Input: part model. Units: mm. Frame: model coordinates. Face numbers are marked on the shaded views. A direction names the side the tool comes from. Coordinates: 2 decimals unless noted, no trailing zeros. Loops run counter-clockwise (first coordinate to the right, second up) from the corner with the lowest first, then second, coordinate; pieces in that order, holes last. Notation, with made-up numbers: (5.5, 41) -> (27.5, 41) arc R26 ccw to (27.5, 73) -> close; hole circle Ø1 at (84.25, -18.75). An arc over 180 degrees is marked (long way). Put each result on its own line as item: value. Start each with the question number.
1) Pull-direction query (Y, two-part tool) for the marked faces 4, 5, 6 and 7; classes: pulls with the +Y half, pulls with the -Y half, needs draft (parallel to the pull), parting line crosses it, or undercut.
2) Cut plane D-D (z = 28). Return the cut outline in (x, y), plus the area to 3 significant figures.
3) Cut plane B-B (x = 0). Return the cut outline in (y, z).
4) Material intervals for L1, parallel to X at y = -2.5, z = 12; L2, parallel to Y at x = 0, z = 4.5; L3, parallel to Z at x = -4.5, y = 9.5, sorted ascending.
5) Set-up query: the marked faces 1, 2 and 3. Return all of +Z, -Z, +X, -X, +Y, -Y with unobstructed straight access to the full face (end or side cutting, diameter ignored); none if empty.
6) Cut plane A-A (z = 22). Return the cut outline in (x, y), plus the area to 3 significant figures.
7) Contact query for flat-ended pins moving along their axis: P1, Ø9, axis at y = 0, z = 32, coming from the -X side; P2, Ø13.5, axis at x = -20.5, z = 21, coming from the -Y side; P3, Ø2, axis at x = 14.5, y = 9.5, coming from the +Z side; P4, Ø2, axis at x = 23, y = -2.5, coming from the +Z side. Output: stop coordinate, or through.
8) Cut plane C-C (y = 6). Return the cut outline in (x, z).
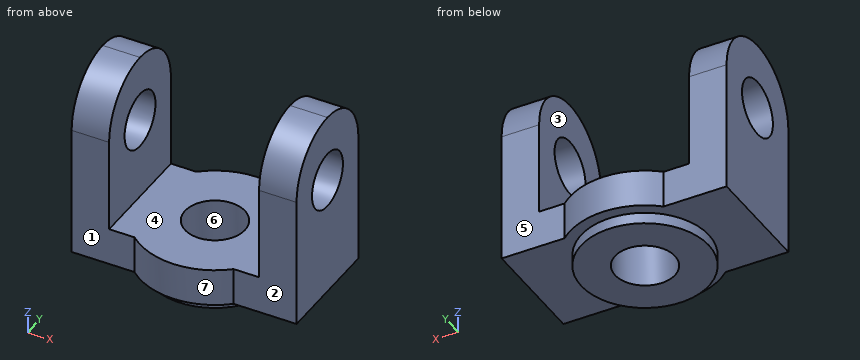
from build123d import *

# Parameters (mm, degrees)
F0_R     = 20
F0_R_2   = 8
F1_DEPTH = 10
F2_R     = 17
F2_R_2   = 8
F3_DEPTH = 3
F5_DEPTH = 15
F6_R     = 8
F7_DEPTH = 25
F8_R     = 7.5
F9_DEPTH = 30


with BuildPart() as f1:
    # F0 (on Top) → F1 (new body)
    with BuildSketch(Plane.XY):
        Circle(F0_R)
        Circle(F0_R_2, mode=Mode.SUBTRACT)
    extrude(amount=F1_DEPTH)

    # F2 (on Top) → F3 (join)
    with BuildSketch(Plane.XY):
        Circle(F2_R)
        Circle(F2_R_2, mode=Mode.SUBTRACT)
    extrude(amount=-F3_DEPTH)

    # F4 (on Front) → F5 (join, symmetric)
    with BuildSketch(Plane.XZ):
        Polygon((-30, 50), (-30, 0), (30, 0), (30, 50), (20, 50), (20, 10), (-20, 10), (-20, 50), align=None)
    extrude(amount=F5_DEPTH, both=True)

    # F6 (on face) → F7 (cut)
    with BuildSketch(Plane.XY.offset(10)):
        Circle(F6_R)
    extrude(amount=-F7_DEPTH, mode=Mode.SUBTRACT)

    # F8 (on Right) → F9 (cut, symmetric)
    with BuildSketch(Plane.YZ):
        with Locations((0, 32)):
            Circle(F8_R)
        with BuildLine():
            ThreePointArc((-15, 35), (-10.606602, 45.606602), (0, 50))
            Line((0, 50), (-15, 50))
            Line((-15, 50), (-15, 35))
        make_face()
        with BuildLine():
            ThreePointArc((0, 50), (10.606602, 45.606602), (15, 35))
            Line((15, 35), (15, 50))
            Line((15, 50), (0, 50))
        make_face()
    extrude(amount=F9_DEPTH, both=True, mode=Mode.SUBTRACT)


solid = f1.part
Results found:
1. face 4: needs draft
1. face 5: pulls with the +Y half
1. face 6: undercut
1. face 7: pulls with the -Y half
2. outline: (-30, -15) -> (-20, -15) -> (-20, -6.34) -> (-30, -6.34) -> close; (-30, 6.34) -> (-20, 6.34) -> (-20, 15) -> (-30, 15) -> close; (20, -15) -> (30, -15) -> (30, -6.34) -> (20, -6.34) -> close; (20, 6.34) -> (30, 6.34) -> (30, 15) -> (20, 15) -> close
2. area: 346 mm2
3. outline: (-20, 0) -> (-17, 0) -> (-17, -3) -> (-8, -3) -> (-8, 10) -> (-20, 10) -> close; (8, -3) -> (17, -3) -> (17, 0) -> (20, 0) -> (20, 10) -> (8, 10) -> close
4. L1: x = -30 to -20, 20 to 30
4. L2: y = -20 to -8, 8 to 20
4. L3: z = -3 to 10
5. face 1: +Z, -Z, -X, -Y
5. face 2: +Z, -Z, +X, -Y
5. face 3: +Z, +Y, -Y
6. outline: (-30, -15) -> (-20, -15) -> (-20, 15) -> (-30, 15) -> close; (20, -15) -> (30, -15) -> (30, 15) -> (20, 15) -> close
6. area: 600 mm2
7. P1: passes through
7. P2: stops at y = -15
7. P3: stops at z = 10
7. P4: stops at z = 49.92
8. outline: (-30, 0) -> (-15.91, 0) -> (-15.91, -3) -> (-5.29, -3) -> (-5.29, 10) -> (-20, 10) -> (-20, 27.5) -> (-30, 27.5) -> close; (-30, 36.5) -> (-20, 36.5) -> (-20, 48.75) -> (-30, 48.75) -> close; (5.29, -3) -> (15.91, -3) -> (15.91, 0) -> (30, 0) -> (30, 27.5) -> (20, 27.5) -> (20, 10) -> (5.29, 10) -> close; (20, 36.5) -> (30, 36.5) -> (30, 48.75) -> (20, 48.75) -> close
